from build123d import *

# Parameters (mm, degrees)
SKETCH1_W           = 190
SKETCH1_H           = 140
BOSS_EXTRUDE1_DEPTH = 5
SKETCH2_W           = 160
SKETCH2_H           = 104
CUT_EXTRUDE1_DEPTH  = 5
SKETCH3_W           = 180
SKETCH3_H           = 130
BOSS_EXTRUDE2_DEPTH = 15
SKETCH4_W           = 170
SKETCH4_H           = 120
CUT_EXTRUDE2_DEPTH  = 10
FILLET1_R           = 0.9
FILLET2_R           = 0.9
SKETCH5_R           = 5.850988458
SKETCH5_W           = 11.444331631
SKETCH5_H           = 13.771992302
CUT_EXTRUDE3_DEPTH  = 10
FILLET3_R           = 5


with BuildPart() as part:
    # Sketch1 → Boss-Extrude1 (new body)
    with BuildSketch(Plane.XY):
        with Locations((-8.247588424, 0.40192926)):
            Rectangle(SKETCH1_W, SKETCH1_H)
    extrude(amount=BOSS_EXTRUDE1_DEPTH)

    # Sketch2 → Cut-Extrude1 (cut)
    with BuildSketch(Plane(origin=(0, 0, 0), x_dir=(-1, 0, 0), z_dir=(0, 0, -1))):
        with Locations((8.247588424, 0.40192926)):
            Rectangle(SKETCH2_W, SKETCH2_H)
    extrude(amount=-CUT_EXTRUDE1_DEPTH, mode=Mode.SUBTRACT)

    # Sketch3 → Boss-Extrude2 (add)
    with BuildSketch(Plane.XY.offset(5)):
        with Locations((-8.247588424, 0.40192926)):
            Rectangle(SKETCH3_W, SKETCH3_H)
    extrude(amount=BOSS_EXTRUDE2_DEPTH)

    # Sketch4 → Cut-Extrude2 (cut)
    with BuildSketch(Plane.XY.offset(20)):
        with Locations((-8.247588424, 0.40192926)):
            Rectangle(SKETCH4_W, SKETCH4_H)
    extrude(amount=-CUT_EXTRUDE2_DEPTH, mode=Mode.SUBTRACT)

    # Fillet1
    fillet1_edges = [part.edges().sort_by_distance(p)[0] for p in [
        (71.752411576, 0.40192926, 0),
        (-8.247588424, -51.59807074, 0),
        (-88.247588424, 0.40192926, 0),
        (-8.247588424, 52.40192926, 0),
    ]]
    fillet(fillet1_edges, radius=FILLET1_R)

    # Fillet2
    fillet2_edges = [part.edges().sort_by_distance(p)[0] for p in [
        (-98.247588424, 65.40192926, 12.5),
        (-98.247588424, -64.59807074, 12.5),
        (81.752411576, -64.59807074, 12.5),
        (81.752411576, 65.40192926, 12.5),
    ]]
    fillet(fillet2_edges, radius=FILLET2_R)

    # Sketch5 → Cut-Extrude3 (cut)
    with BuildSketch(Plane(origin=(0, 0, 5), x_dir=(-1, 0, 0), z_dir=(0, 0, -1))):
        with Locations((-28.456331926, 0)):
            Circle(SKETCH5_R)
        with Locations((1.51229921, -3.046296959)):
            Rectangle(SKETCH5_W, SKETCH5_H)
    extrude(amount=-CUT_EXTRUDE3_DEPTH, mode=Mode.SUBTRACT)

    # Fillet3
    fillet3_edges = [part.edges().sort_by_distance(p)[0] for p in [
        (-103.247588424, 70.40192926, 2.5),
        (86.752411576, 70.40192926, 2.5),
        (86.752411576, -69.59807074, 2.5),
        (-103.247588424, -69.59807074, 2.5),
    ]]
    fillet(fillet3_edges, radius=FILLET3_R)


solid = part.part
Geometry: final body of the model. Coordinates: model frame, mm. A direction names the side the tool comes from. Round coordinates to 2 decimals unless told otherwise and drop trailing zeros. Write each loop counter-clockwise with the first axis right and the second up, starting at its lowest first coordinate (ties: lowest second). Pieces come first, ordered by that corner, then holes. Notation, with made-up numbers: M -1,-2 L 57,-2 A25 ccw 57,31 Z; hole C 81,16 d1. An arc over 180 degrees is marked long. Write item = value, one per line.
Item 1: Material intervals for line 1 along Y through (x, z) = (-92, 12); line 2 along X through (y, z) = (-7.5, 17.25); line 3 along X through (y, z) = (-19.5, 1), sorted ascending. Write a range as [from, to].
Findings:
line_1 = [-64.6, -59.6], [60.4, 65.4]
line_2 = [-98.25, -93.25], [76.75, 81.75]
line_3 = [-103.25, -88.25], [71.75, 86.75]
Item 2: Pin query (flat end, axial travel): P1, Ø3, axis at y = -4, z = 15, coming from the -X side; P2, Ø12, axis at y = 17, z = 10, coming from the -X side; P3, Ø1.5, axis at x = -1.5, z = 7.5, coming from the -Y side; P4, Ø1.5, axis at y = -6.5, z = 8, coming from the +X side. Return the tip coordinate at first contact, or that it passes through.
Findings:
P1 = -98.25
P2 = -103.25
P3 = -64.6
P4 = 81.75
Item 3: Access query for faces 1 (the face through (-7, -51.598, 3)), 2 (the face through (-9, 1, 10)), 3 (the face through (-9, 65.402, 12)). Directions: +Z, -Z, +X, -X, +Y, -Y. A direction counts if a zero-diameter tool reaches every point of the face in a straight line with its end or side. Return the directions, or none.
Findings:
face_1 = -Z
face_2 = +Z
face_3 = +Z, +X, -X, +Y
Item 4: Section query B-B on x = 0.5. Return loops of the section in (y, z), then the cut area to 3 significant figures.
Findings:
outline = M -69.6,0 L -52.5,0 A0.9 ccw -51.6,0.9 L -51.6,5 L -9.93,5 L -9.93,10 L -59.6,10 L -59.6,20 L -64.6,20 L -64.6,5 L -69.6,5 Z; M 3.84,5 L 52.4,5 L 52.4,0.9 A0.9 ccw 53.3,0 L 70.4,0 L 70.4,5 L 65.4,5 L 65.4,20 L 60.4,20 L 60.4,10 L 3.84,10 Z
area = 861 mm^2
Item 5: Section query C-C on z = 15. Return loops of the section in (x, y).
Findings:
outline = M -98.25,-63.7 A0.9 ccw -97.35,-64.6 L 80.85,-64.6 A0.9 ccw 81.75,-63.7 L 81.75,64.5 A0.9 ccw 80.85,65.4 L -97.35,65.4 A0.9 ccw -98.25,64.5 Z; hole M -93.25,-59.6 L 76.75,-59.6 L 76.75,60.4 L -93.25,60.4 Z
Item 6: Section query A-A on y = 0. Return loops of the section in (x, z), then the cut area to 3 significant figures.
Findings:
outline = M -103.25,0 L -89.15,0 A0.9 ccw -88.25,0.9 L -88.25,5 L -7.23,5 L -7.23,10 L -93.25,10 L -93.25,20 L -98.25,20 L -98.25,5 L -103.25,5 Z; M 4.21,5 L 22.61,5 L 22.61,10 L 4.21,10 Z; M 34.31,5 L 71.75,5 L 71.75,0.9 A0.9 ccw 72.65,0 L 86.75,0 L 86.75,5 L 81.75,5 L 81.75,20 L 76.75,20 L 76.75,10 L 34.31,10 Z
area = 1,030 mm^2
Item 7: Section query D-D on x = -56. Return loops of the section in (y, z).
Findings:
outline = M -69.6,0 L -52.5,0 A0.9 ccw -51.6,0.9 L -51.6,5 L 52.4,5 L 52.4,0.9 A0.9 ccw 53.3,0 L 70.4,0 L 70.4,5 L 65.4,5 L 65.4,20 L 60.4,20 L 60.4,10 L -59.6,10 L -59.6,20 L -64.6,20 L -64.6,5 L -69.6,5 Z
Item 8: Pull-direction query (X, two-part tool) for faces 4 (the face through (85.249, 68.976, 2.535)), 5 (the face through (-9, 60.402, 15)), 6 (the face through (-9, -64.598, 12)), 7 (the face through (-1, -9.932, 7)); classes: pulls with the +X half, pulls with the -X half, needs draft (parallel to the pull), parting line crosses it, or undercut.
Findings:
face_4 = pulls with the +X half
face_5 = undercut
face_6 = needs draft
face_7 = undercut
